```python
from build123d import *

# Parameters (mm, degrees)
RESSALTO_EXTRUS_O1_DEPTH = 6
CORTE_EXTRUS_O2_DEPTH    = 76


with BuildPart() as part:
    # Model → Ressalto-extrusão1 (new body)
    with BuildSketch(Plane.XY):
        Polygon((35, -42.315), (35, -54.735), (-35, -54.735), (-35, -42.315), (-40, -42.315), (-40, -32.465), (-35, -32.465), (-35, -28.965000001), (-27, -28.965000001), (-27, -30.965000001), (-22, -30.965000001), (-22, -23.965000001), (-27, -23.965000001), (-27, -25.965000001), (-35, -25.965000001), (-35, -22.265), (-40, -22.265), (-40, -12.415), (-35, -12.415), (-35, 0), (35, 0), (35, -12.415), (40, -12.415), (40, -22.265), (35, -22.265), (35, -25.965000001), (27, -25.965000001), (27, -23.965000001), (22, -23.965000001), (22, -30.965000001), (27, -30.965000001), (27, -28.965000001), (35, -28.965000001), (35, -32.465), (40, -32.465), (40, -42.315), align=None)
    extrude(amount=RESSALTO_EXTRUS_O1_DEPTH)

    # Esboço2 → Corte-extrusão2 (cut, through all)
    with BuildSketch(Plane(origin=(35, 0, 0), x_dir=(0, 0, -1), z_dir=(1, 0, 0))):
        Polygon((-6, -0.75), (0, -5.75), (0, 4.25), (-6, 4.25), align=None)
        Polygon((-6, -58.99), (-6, -53.99), (0, -48.99), (0, -58.99), align=None)
    extrude(amount=-CORTE_EXTRUS_O2_DEPTH, mode=Mode.SUBTRACT)


solid = part.part
```
Check sheet for the modelled part. Datum: model origin and axes. Units: mm. A direction names the side the tool comes from. Round coordinates to 2 decimals unless told otherwise and drop trailing zeros. Order: outer loops, then holes, each group sorted by start corner. A loop starts at its lowest first (then second) coordinate and runs counter-clockwise, first axis right, second up. Notation, with made-up numbers: (-33, 79.25) -> (12, 79.25) arc R28 ccw to (12, 114.25) -> close; hole circle Ø11 at (4, 37). An arc over 180 degrees is marked (long way). One line per item, written item: value. Start each with the question number.
Q1. Mould release check, pull along X, two halves, no side actions. Record for faces 4 (the face through (22, -27, 3)), 5 (the face through (35, -8, 3)), 6 (the face through (38, -22.265, 3)), 7 (the face through (-35, -47, 3)): pulls with the +X half, pulls with the -X half, needs draft (parallel to the pull), parting line crosses it, or undercut.
Q2. Set-up check for faces 1 (the face through (-27, -30, 3)), 2 (the face through (-37, -22.265, 3)), 3 (the face through (37, -12.415, 3)): record each of +Z, -Z, +X, -X, +Y, -Y from which the full face is reachable in a straight line by a thin tool's end or side.
Q3. Cross-section at C-C (y = -9). Record the boundary of the cut face in (x, z).
Q4. Thickness scan on line 1 (X direction, y = -29, z = 1.35); line 2 (Y direction, x = 37, z = 4.35) (3 decimals); line 3 (Y direction, x = -24.5, z = 1.6) (3 decimals). Record the ranges inside material, lowest first.
Q5. Cross-section at D-D (x = -6.5). Record the boundary of the cut face in (y, z).
Q6. Gauge pin test, flat ends, axial feed: pin 1 Ø1.8 at (y, z) = (-45.5, 3) entering from +X; pin 2 Ø1.5 at (x, z) = (-37.5, 2.5) entering from +Y (3 decimals); pin 3 Ø3 at (x, z) = (30.5, 2.5) entering from +Y. Record the tip position at first contact, or that the pin passes through.
Q7. Cross-section at B-B (x = 32). Record the boundary of the cut face in (y, z) (3 decimals).
Q8. Cross-section at A-A (x = 24). Record the boundary of the cut face in (y, z) (3 decimals).
Completed:
1. face 4: undercut
1. face 5: pulls with the +X half
1. face 6: needs draft
1. face 7: pulls with the -X half
2. face 1: +Z, -Z
2. face 2: +Z, -Z, -X
2. face 3: +Z, -Z, +X, +Y
3. outline: (-35, 0) -> (35, 0) -> (35, 6) -> (-35, 6) -> close
4. line 1: x = -35 to -27, -22 to 22, 27 to 35
4. line 2: y = -42.315 to -32.465, -22.265 to -12.415
4. line 3: y = -50.323 to -30.965, -23.965 to -4.417
5. outline: (-53.99, 6) -> (-48.99, 0) -> (-5.75, 0) -> (-0.75, 6) -> close
6. pin 1: stops at x = 35
6. pin 2: stops at y = -12.415
6. pin 3: stops at y = -2.42
7. outline: (-53.99, 6) -> (-48.99, 0) -> (-28.965, 0) -> (-28.965, 6) -> close; (-25.965, 0) -> (-5.75, 0) -> (-0.75, 6) -> (-25.965, 6) -> close
8. outline: (-53.99, 6) -> (-48.99, 0) -> (-30.965, 0) -> (-30.965, 6) -> close; (-23.965, 0) -> (-5.75, 0) -> (-0.75, 6) -> (-23.965, 6) -> close
